Can you work these out from the model? Positions are in its coordinate system, mm. Face numbers are marked on the shaded views. Round coordinates to 2 decimals unless told otherwise and drop trailing zeros. Loops run counter-clockwise (first coordinate to the right, second up) from the corner with the lowest first, then second, coordinate; pieces in that order, holes last.
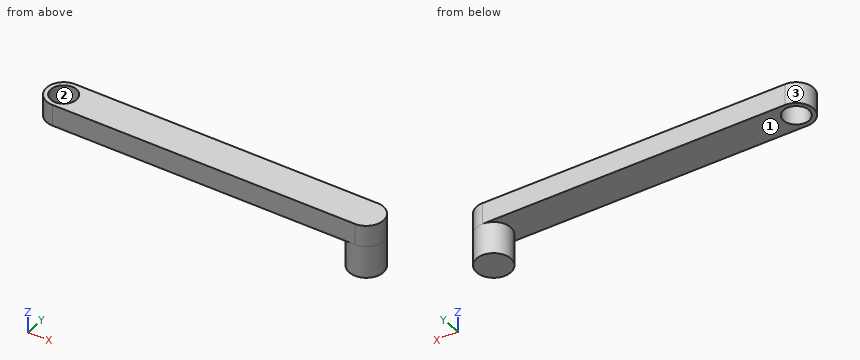
from build123d import *

# Parameters (mm, degrees)
SKETCH1_R           = 8
SKETCH1_R_2         = 6
BOSS_EXTRUDE1_DEPTH = 10
SKETCH1_6_R         = 8
BOSS_EXTRUDE2_DEPTH = 15


with BuildPart() as part:
    # Sketch1 → Boss-Extrude1 (new body)
    with BuildSketch(Plane.XY):
        with BuildLine():
            Line((190, 8), (50, 8))
            ThreePointArc((50, 8), (55.656854249, 5.656854249), (58, 0))
            ThreePointArc((58, 0), (55.656854249, -5.656854249), (50, -8))
            Line((50, -8), (190, -8))
            ThreePointArc((190, -8), (182, 0), (190, 8))
        make_face()
        with Locations((50, 0)):
            Circle(SKETCH1_R)
        with Locations((50, 0)):
            Circle(SKETCH1_R_2, mode=Mode.SUBTRACT)
        with Locations((190, 0)):
            Circle(SKETCH1_R)
    extrude(amount=BOSS_EXTRUDE1_DEPTH)

    # Sketch1_6 → Boss-Extrude2 (add)
    with BuildSketch(Plane.XY):
        with Locations((190, 0)):
            Circle(SKETCH1_6_R)
    extrude(amount=-BOSS_EXTRUDE2_DEPTH)


solid = part.part
(1) If we mould it in two halves opening along Y, with no side actions, what happens to the marked faces 1, 2 and 3? For each: released by +Y, released by -Y, zero draft, split by the parting line, or undercut.
Worked answers:
face 1: zero draft
face 2: undercut
face 3: split by the parting line
(2) Will these pins go through, and if not, where does the flat tip stop? P1, Ø4, axis at y = 6, z = -5, coming from the -X side; P2, Ø8, axis at x = 150.5, y = -4, coming from the -Z side.
Worked answers:
P1: stops at x = 183.07
P2: stops at z = 0
(3) If I drill on line 1 (Y direction, x = 50, z = 4.75); line 2 (Z direction, x = 156.5, y = -1.5); line 3 (X direction, y = 3.25, z = 7.5), over which ranges is the centre line in solid material (lowest first)?
Worked answers:
line 1: y = -8 to -6, 6 to 8
line 2: z = 0 to 10
line 3: x = 42.69 to 44.96, 55.04 to 197.31
(4) If we section it at A-A, the plane z = 3: List the corners of the cut face in (x, y) for me.
Worked answers:
outline: (50, -8) - (190, -8) arc R8 ccw to (190, 8) - (50, 8) arc R8 ccw to start; hole circle Ø12 at (50, 0)
(5) If we section it at B-B, the plane y = 0: List the corners of the cut face in (x, z) for me.
Worked answers:
outline: (42, 0) - (44, 0) - (44, 10) - (42, 10) - close; (56, 0) - (182, 0) - (182, -15) - (198, -15) - (198, 10) - (56, 10) - close
(6) If we section it at D-D, the plane z = -11.25: List the corners of the cut face in (x, y) for me.
Worked answers:
outline: circle Ø16 at (190, 0)
(7) If we section it at C-C, the plane x = 166: List the corners of the cut face in (y, z) for me.
Worked answers:
outline: (-8, 0) - (8, 0) - (8, 10) - (-8, 10) - close
